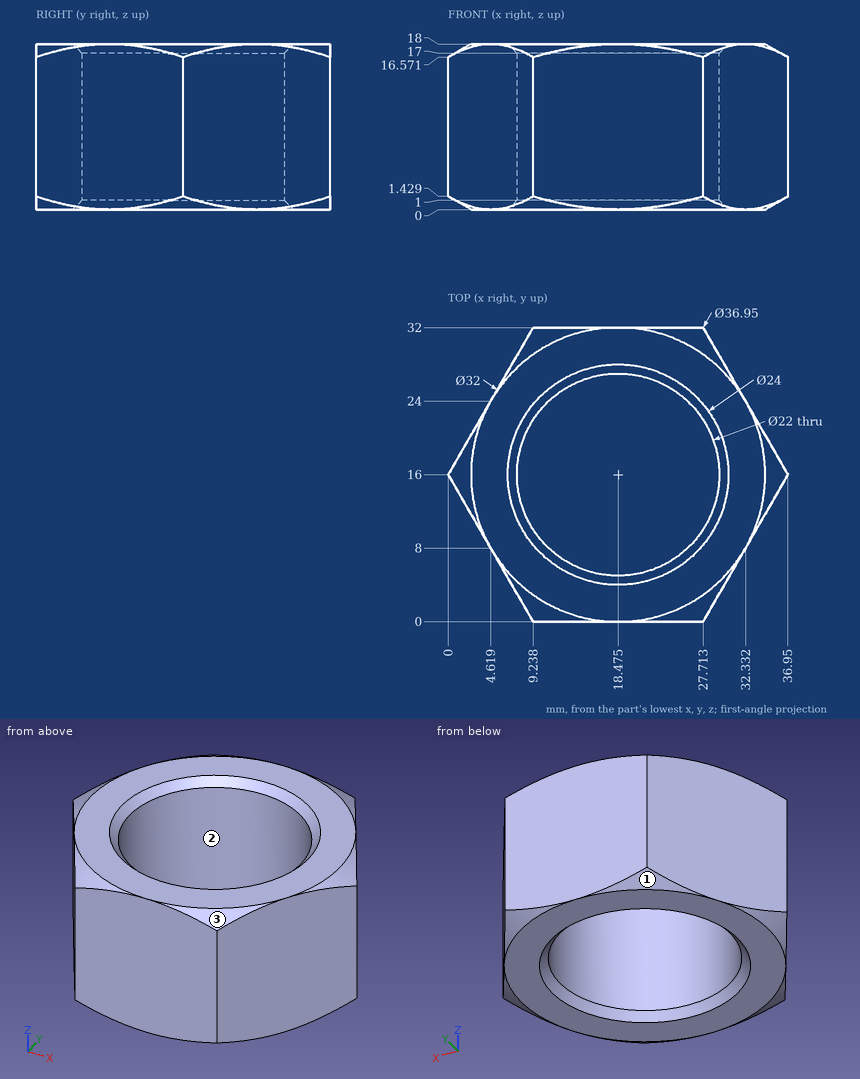
The drawing under review shows one solid part. Ordinate dimensions are in mm from its lowest x, y, z. Round coordinates to 2 decimals unless told otherwise and drop trailing zeros. Answer in a Markdown table with one row per item.
1) Draft analysis for pull direction X (two halves, no side actions). For the marked faces 1, 2 and 3, state which applies: pulls with the +X half, pulls with the -X half, needs draft (parallel to the pull), parting line crosses it, or undercut.
Taken from the geometry:
| item | result |
|---|---|
| face 1 | pulls with the -X half |
| face 2 | undercut |
| face 3 | pulls with the +X half |
2) Wall thickness on line 1 along Y through (x, z) = (18, 4.25); line 2 along X through (y, z) = (9, 13.25); line 3 along X through (y, z) = (16.5, 2) (1 decimal): over which ranges is each line inside the solid? List them lowest first.
Taken from the geometry:
| item | result |
|---|---|
| line 1 | y = 0 to 5.01, 26.99 to 32 |
| line 2 | x = 4.04 to 9.99, 26.96 to 32.91 |
| line 3 | x = 0.3 to 7.5, 29.5 to 36.7 |
3) For pin 1 Ø1 at (x, z) = (8.5, 5.5) entering from -Y; pin 2 Ø8 at (y, z) = (24, 11.5) entering from -X; pin 3 Ø13 at (x, y) = (18.48, 16) entering from -Z; pin 4 Ø2 at (y, z) = (15.5, 2.5) entering from +X, all flat-tipped, find the tip position at first contact; note any pin that passes through.
Taken from the geometry:
| item | result |
|---|---|
| pin 1 | stops at y = 0.41 |
| pin 2 | stops at x = 2.31 |
| pin 3 | passes through |
| pin 4 | stops at x = 36.95 |
